Check sheet for the modelled part. Datum: model origin and axes. Units: mm. Face numbers are marked on the shaded views. Round coordinates to 2 decimals unless told otherwise and drop trailing zeros. Loops run counter-clockwise (first coordinate to the right, second up) from the corner with the lowest first, then second, coordinate; pieces in that order, holes last. Notation, with made-up numbers: M 9,9 L 64,9 A17 cw 64,40 Z; hole C 48,-27.75 d11. An arc over 180 degrees is marked long. Write item = value, one per line. Start each with the question number.
(1) Cross-section at D-D on z = 1.15. Record the boundary of the cut face in (x, y), plus the area to 3 significant figures.
(2) Cross-section at A-A on y = -8. Record the boundary of the cut face in (x, z).
(3) Mould release check, pull along Y, two halves, no side actions. Record for the marked faces 1, 2, 3 and 4: pulls with the +Y half, pulls with the -Y half, needs draft (parallel to the pull), parting line crosses it, or undercut.
(4) Scan lines: L1, parallel to Z at x = 2.5, y = 2; L2, parallel to Y at x = 5, z = -0.8; L3, parallel to X at y = -2.5, z = -1.15. Record each from-to range of solid material in increasing order. Write a range as from..to.
(5) Cross-section at C-C on y = -0.75. Record the boundary of the cut face in (x, z), plus the area to 3 significant figures.
(6) Go/stop test with flat-tipped pins: P1, Ø4, axis at x = -4.5, y = -3.5, coming from the +Z side; P2, Ø1.5, axis at x = -7, z = -2, coming from the -Y side; P3, Ø0.7, axis at x = -10, z = -1.5, coming from the -Y side. Record where each tip stops, or that it passes through.
(7) Cross-section at B-B on x = 2. Record the boundary of the cut face in (y, z).
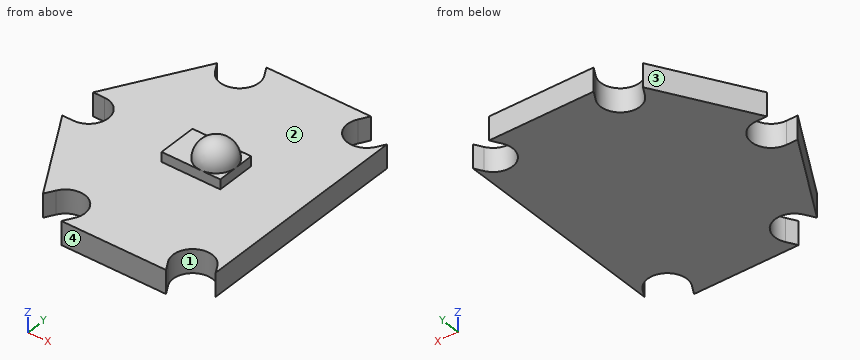
Autodesk Inventor part; units mm, degrees
ref_plane "YZ Plane" through (0, 0, 0) normal (1, 0, 0) x (0, 1, 0)
ref_plane "XZ Plane" through (0, 0, 0) normal (0, 1, 0) x (-1, 0, 0)
ref_plane "XY Plane" through (0, 0, 0) normal (0, 0, 1) x (1, 0, 0)
sketch "Skizze1" plane through (0, 0, 0) normal (0, 0, 1) x (1, 0, 0)
  line L0 (-3, 1.5) -> (1.5, 1.5)
  line L1 (1.5, 1.5) -> (1.5, -1.5)
  line L2 (-3, -1.5) -> (-3, 1.5)
  line L3 (1.5, 1.5) -> (-1.5, -1.5) construction
  line L4 (-1.5, -1.5) -> (1.5, -1.5) construction
  line L5 (0, 0) -> (0.1963, -0.4081) construction
  line L6 (-3, -1.5) -> (1.5, -1.5)
  dimension "d0" = 3
  dimension "d1" = 4.5
extrude "Extrusion1" add sketch "Skizze1" against normal blind 0.75
sketch "Skizze2" plane through (0, 0, 0) normal (1, 0, 0) x (0, 1, 0)
  line L0 (-1.5, 0) -> (1.5, 0)
  arc A0 (0, 1.5) -> (-1.5, 0) centre (0, 0) ccw
  line L1 (0, 0) -> (0, 1.5)
  line L2 (0, 0) -> (-1.5, 0)
  dimension "d4" = 1.5
revolve "Umdrehung1" add sketch "Skizze2" angle 360 about axis through (0, 0, 0) along (0, 0, 1)
sketch "Skizze3" plane through (0, 0, -0.75) normal (0, 0, -1) x (-1, 0, 0)
  line L0 (11.4893, 0) -> (5.7446, -9.95)
  line L1 (5.7446, -9.95) -> (-5.7446, -9.95)
  line L2 (-5.7446, -9.95) -> (-11.4893, 0)
  line L3 (-11.4893, 0) -> (-5.7446, 9.95)
  line L4 (-5.7446, 9.95) -> (5.7446, 9.95)
  line L5 (5.7446, 9.95) -> (11.4893, 0)
  point P0 (0, 0)
  point P1 (0, 0)
  dimension "d7" = 19.9
extrude "Extrusion2" add sketch "Skizze3" along normal blind 1.8
sketch "Skizze4" plane through (0, 0, -0.75) normal (0, 0, 1) x (1, 0, 0)
  line L0 (-11.4893, 0) -> (-5.7446, -9.95)
  line L1 (-5.7446, 9.95) -> (-11.4893, 0)
  line L2 (1.5, -1.5) -> (-3, -1.5)
  line L3 (0, 0) -> (-9.77, 0) construction
  arc A0 (-9.77, -1.5) -> (-9.77, 1.5) centre (-9.77, 0) ccw
  line L4 (-9.77, -1.5) -> (-10.6232, -1.5)
  line L5 (-9.77, 1.5) -> (-10.6232, 1.5)
  dimension "d10" = 9.77
  dimension "d11" = 3
extrude "Extrusion3" cut sketch "Skizze4" against normal blind 1.8
pattern_circular "Runde Anordnung1" count 6 over 360 about axis through (0, 0, -10) along (0, 0, 1) of "Extrusion3"
ref_plane "Arbeitsebene1" through (13.7343, 6, -7.9495) normal (0.7071068, 0, 0.7071068) x (0, 1, 0)
sketch "Skizze6" plane through (0, 0, -0.75) normal (0, 0, 1) x (1, 0, 0)
  line L0 (-6.184, 7.7111) -> (-6.6107, 8.45) construction
  line L1 (-6.6107, 8.45) -> (-10.6232, 1.5) construction
  line L2 (-10.6232, 1.5) -> (-9.77, 1.5) construction
  arc A0 (-9.77, -1.5) -> (-9.77, 1.5) centre (-9.77, 0) ccw construction
  line L3 (-9.77, -1.5) -> (-10.6232, -1.5) construction
  line L4 (-10.6232, -1.5) -> (-6.6107, -8.45) construction
  line L5 (-6.6107, -8.45) -> (-6.184, -7.7111) construction
  arc A1 (-3.586, -9.2111) -> (-6.184, -7.7111) centre (-4.885, -8.4611) ccw construction
  line L6 (-3.586, -9.2111) -> (-4.0126, -9.95) construction
  line L7 (-4.0126, -9.95) -> (4.0126, -9.95) construction
  line L8 (4.0126, -9.95) -> (3.586, -9.2111) construction
  arc A2 (6.184, -7.7111) -> (3.586, -9.2111) centre (4.885, -8.4611) ccw construction
  line L9 (6.184, -7.7111) -> (6.6107, -8.45) construction
  line L10 (6.6107, -8.45) -> (10.6232, -1.5)
  line L11 (10.6232, -1.5) -> (9.77, -1.5)
  arc A3 (9.77, 1.5) -> (9.77, -1.5) centre (9.77, 0) ccw
  line L12 (9.77, 1.5) -> (10.6232, 1.5)
  line L13 (10.6232, 1.5) -> (6.6107, 8.45)
  line L14 (6.6107, 8.45) -> (6.184, 7.7111) construction
  arc A4 (3.586, 9.2111) -> (6.184, 7.7111) centre (4.885, 8.4611) ccw construction
  line L15 (3.586, 9.2111) -> (4.0126, 9.95) construction
  line L16 (4.0126, 9.95) -> (-4.0126, 9.95) construction
  line L17 (-4.0126, 9.95) -> (-3.586, 9.2111) construction
  arc A5 (-6.184, 7.7111) -> (-3.586, 9.2111) centre (-4.885, 8.4611) ccw construction
  line L18 (-3, -1.5) -> (-3, 1.5) construction
  line L19 (-3, 1.5) -> (1.5, 1.5) construction
  line L20 (1.5, 1.5) -> (1.5, -1.5) construction
  line L21 (1.5, -1.5) -> (-3, -1.5) construction
  line L22 (-4.0126, -9.95) -> (-3.586, -9.2111) construction
  arc A6 (-3.586, -9.2111) -> (-6.184, -7.7111) centre (-4.885, -8.4611) ccw construction
  line L23 (-6.184, -7.7111) -> (-6.6107, -8.45) construction
  line L24 (-6.6107, -8.45) -> (-10.6232, -1.5) construction
  line L25 (-10.6232, -1.5) -> (-9.77, -1.5) construction
  arc A7 (-9.77, -1.5) -> (-9.77, 1.5) centre (-9.77, 0) ccw construction
  line L26 (-9.77, 1.5) -> (-10.6232, 1.5) construction
  line L27 (-10.6232, 1.5) -> (-6.6107, 8.45) construction
  line L28 (-6.6107, 8.45) -> (-6.184, 7.7111) construction
  arc A8 (-6.184, 7.7111) -> (-3.586, 9.2111) centre (-4.885, 8.4611) ccw construction
  line L29 (-3.586, 9.2111) -> (-4.0126, 9.95) construction
  line L30 (-4.0126, 9.95) -> (4.0126, 9.95) construction
  line L31 (4.0126, 9.95) -> (3.586, 9.2111) construction
  arc A9 (3.586, 9.2111) -> (6.184, 7.7111) centre (4.885, 8.4611) ccw construction
  line L32 (6.184, 7.7111) -> (6.6107, 8.45) construction
  line L33 (6.6107, 8.45) -> (10.6232, 1.5) construction
  line L34 (10.6232, 1.5) -> (9.77, 1.5)
  arc A10 (9.77, 1.5) -> (9.77, -1.5) centre (9.77, 0) ccw
  line L35 (9.77, -1.5) -> (10.6232, -1.5)
  line L36 (10.6232, -1.5) -> (6.6107, -8.45) construction
  line L37 (6.6107, -8.45) -> (6.184, -7.7111) construction
  arc A11 (6.184, -7.7111) -> (3.586, -9.2111) centre (4.885, -8.4611) ccw construction
  line L38 (3.586, -9.2111) -> (4.0126, -9.95) construction
  line L39 (4.0126, -9.95) -> (-4.0126, -9.95) construction
  line L40 (-3, -1.5) -> (-3, 1.5) construction
  line L41 (-3, 1.5) -> (1.5, 1.5) construction
  line L42 (1.5, 1.5) -> (1.5, -1.5) construction
  line L43 (1.5, -1.5) -> (-3, -1.5) construction
  line L44 (-4.0126, -9.95) -> (-3.586, -9.2111) construction
  arc A12 (-3.586, -9.2111) -> (-6.184, -7.7111) centre (-4.885, -8.4611) ccw construction
  line L45 (-6.184, -7.7111) -> (-6.6107, -8.45) construction
  line L46 (-6.6107, -8.45) -> (-10.6232, -1.5) construction
  line L47 (-10.6232, -1.5) -> (-9.77, -1.5) construction
  arc A13 (-9.77, -1.5) -> (-9.77, 1.5) centre (-9.77, 0) ccw construction
  line L48 (-9.77, 1.5) -> (-10.6232, 1.5) construction
  line L49 (-10.6232, 1.5) -> (-6.6107, 8.45) construction
  line L50 (-6.6107, 8.45) -> (-6.184, 7.7111) construction
  arc A14 (-6.184, 7.7111) -> (-3.586, 9.2111) centre (-4.885, 8.4611) ccw construction
  line L51 (-3.586, 9.2111) -> (-4.0126, 9.95) construction
  line L52 (-4.0126, 9.95) -> (4.0126, 9.95) construction
  line L53 (4.0126, 9.95) -> (3.586, 9.2111) construction
  arc A15 (3.586, 9.2111) -> (6.184, 7.7111) centre (4.885, 8.4611) ccw construction
  line L54 (6.184, 7.7111) -> (6.6107, 8.45) construction
  line L55 (6.6107, 8.45) -> (10.6232, 1.5) construction
  line L56 (10.6232, 1.5) -> (9.77, 1.5)
  arc A16 (9.77, 1.5) -> (9.77, -1.5) centre (9.77, 0) ccw
  line L57 (9.77, -1.5) -> (10.6232, -1.5)
  line L58 (10.6232, -1.5) -> (6.6107, -8.45) construction
  line L59 (6.6107, -8.45) -> (6.184, -7.7111) construction
  arc A17 (6.184, -7.7111) -> (3.586, -9.2111) centre (4.885, -8.4611) ccw construction
  line L60 (3.586, -9.2111) -> (4.0126, -9.95) construction
  line L61 (4.0126, -9.95) -> (-4.0126, -9.95) construction
  line L62 (-3, -1.5) -> (-3, 1.5) construction
  line L63 (-3, 1.5) -> (1.5, 1.5) construction
  line L64 (1.5, 1.5) -> (1.5, -1.5) construction
  line L65 (1.5, -1.5) -> (-3, -1.5) construction
  line L66 (6.5349, 13.93) -> (6.5349, -13.93) construction
  line L67 (6.6107, -8.45) -> (10.6232, -1.5)
  line L68 (6.6107, -8.45) -> (6.5349, -8.3187)
  line L69 (6.184, -7.7111) -> (6.6107, -8.45)
  line L70 (6.5349, -8.3187) -> (6.5349, 8.3187)
  line L71 (6.6107, 8.45) -> (6.184, 7.7111)
  line L72 (6.5349, 8.3187) -> (6.6107, 8.45)
  point P0 (0, 0)
extrude "Extrusion4" cut sketch "Skizze6" against normal through all
properties part number "Luxeon Rebel Star"
Result:
q1.outline = C 0,0 d1.93
q1.area = 2.91 mm^2
q2.outline = M -6.87,-2.55 L -6.35,-2.55 L -6.35,-0.75 L -6.87,-0.75 Z; M -3.46,-2.55 L 3.46,-2.55 L 3.46,-0.75 L -3.46,-0.75 Z; M 6.35,-2.55 L 6.53,-2.55 L 6.53,-0.75 L 6.35,-0.75 Z
q3.face_1 = undercut
q3.face_2 = needs draft
q3.face_3 = pulls with the +Y half
q3.face_4 = pulls with the -Y half
q4.L1 = -2.55..-0.75
q4.L2 = -6.97..6.97
q4.L3 = -10.05..6.53
q5.outline = M -8.47,-2.55 L 6.53,-2.55 L 6.53,-0.75 L 1.5,-0.75 L 1.5,0 L 1.3,0 A1.3 ccw -1.3,0 L -3,0 L -3,-0.75 L -8.47,-0.75 Z
q5.area = 33.0 mm^2
q6.P1 = -0.75
q6.P2 = -8.45
q6.P3 = -3.19
q7.outline = M -9.95,-2.55 L 9.95,-2.55 L 9.95,-0.75 L -9.95,-0.75 Z
